Check sheet for the modelled part. Datum: model origin and axes. Units: mm. Face numbers are marked on the shaded views. A direction names the side the tool comes from. Coordinates: 2 decimals unless noted, no trailing zeros. Order: outer loops, then holes, each group sorted by start corner. A loop starts at its lowest first (then second) coordinate and runs counter-clockwise, first axis right, second up.
1. Draft check along X on the marked faces 1, 2 and 3. Enter one of: released by +X, released by -X, zero draft, split by the parting line, or undercut.
2. Cross-section at A-A (y = 0). Enter the section's corners in (x, z).
3. Thickness scan on line 1 (Y direction, x = 0, z = 8.25); line 2 (Y direction, x = 0.5, z = 1.25); line 3 (Z direction, x = 0.75, y = 1.9). Record the ranges inside material, lowest first.
4. Cross-section at B-B (x = 0). Enter the section's corners in (y, z).
5. Gauge pin test, flat ends, axial feed: pin 1 Ø1 at (y, z) = (-1, 4) entering from +X; pin 2 Ø0.6 at (y, z) = (-1.5, 0) entering from +X; pin 3 Ø0.5 at (x, y) = (0, 2) entering from -Z; pin 4 Ø1.6 at (x, y) = (0, 0) entering from +Z. Record the tip position at first contact, or that the pin passes through.
6. Cross-section at D-D (z = 9.5). Enter the section's corners in (x, y).
7. Cross-section at C-C (z = 1.5). Enter the section's corners in (x, y), then the cut area to 3 significant figures.
8. Set-up check for the marked faces 4 and 5: record each of +Z, -Z, +X, -X, +Y, -Y from which the full face is reachable in a straight line by a thin tool's end or side.
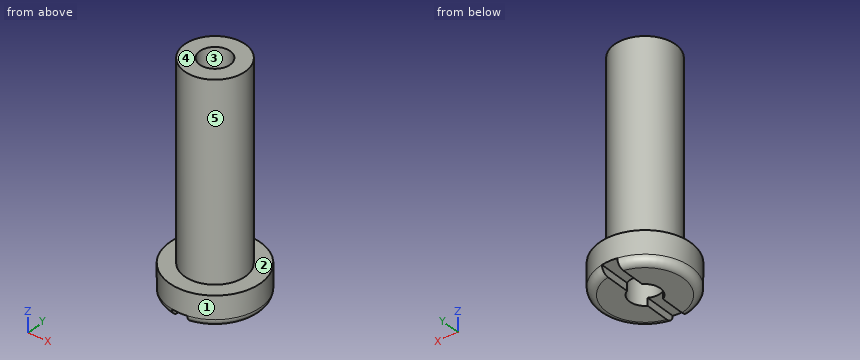
```python
from build123d import *

# Parameters (mm, degrees)
SKETCH1_R               = 3
BOSS_EXTRUDE1_DEPTH     = 2
FILLET1_R               = 0.5
SKETCH2_R               = 2
BOSS_EXTRUDE2_DEPTH     = 12.75
CUT_EXTRUDE1_DEPTH      = 16.348045478
CUT_EXTRUDE1_DEPTH_BACK = 16.348045478
SKETCH3_R               = 1
SKETCH4_W               = 1
SKETCH4_H               = 6
CUT_EXTRUDE3_DEPTH      = 0.5


with BuildPart() as part:
    # Sketch1 → Boss-Extrude1 (new body)
    with BuildSketch(Plane.XY):
        Circle(SKETCH1_R)
    extrude(amount=BOSS_EXTRUDE1_DEPTH)

    # Fillet1
    fillet1_edges = [part.edges().sort_by_distance(p)[0] for p in [
        (-3, 0, 0),
    ]]
    fillet(fillet1_edges, radius=FILLET1_R)

    # Sketch2 → Boss-Extrude2 (add)
    with BuildSketch(Plane.XY.offset(2)):
        Circle(SKETCH2_R)
    extrude(amount=BOSS_EXTRUDE2_DEPTH)

    # Sketch3 → Cut-Extrude1 (cut, two sides: drawn at the far end of the back side and taken through both)
    with BuildSketch(Plane(origin=(0, 0, 0), x_dir=(-1, 0, 0), z_dir=(0, 0, -1)).offset(-CUT_EXTRUDE1_DEPTH_BACK)):
        Circle(SKETCH3_R)
    extrude(amount=CUT_EXTRUDE1_DEPTH + CUT_EXTRUDE1_DEPTH_BACK, mode=Mode.SUBTRACT)

    # Sketch4 → Cut-Extrude3 (cut)
    with BuildSketch(Plane(origin=(0, 0, 0), x_dir=(-1, 0, 0), z_dir=(0, 0, -1))):
        Rectangle(SKETCH4_W, SKETCH4_H)
    extrude(amount=-CUT_EXTRUDE3_DEPTH, mode=Mode.SUBTRACT)


solid = part.part
```
Data:
1. face 1: split by the parting line
1. face 2: zero draft
1. face 3: undercut
2. outline: (-3, 0.5) arc R0.5 ccw to (-2.5, 0) - (-1, 0) - (-1, 14.75) - (-2, 14.75) - (-2, 2) - (-3, 2) - close; (1, 0) - (2.5, 0) arc R0.5 ccw to (3, 0.5) - (3, 2) - (2, 2) - (2, 14.75) - (1, 14.75) - close
3. line 1: y = -2 to -1, 1 to 2
3. line 2: y = -2.96 to -0.87, 0.87 to 2.96
3. line 3: z = 0 to 2
4. outline: (-3, 0.5) - (-1, 0.5) - (-1, 14.75) - (-2, 14.75) - (-2, 2) - (-3, 2) - close; (1, 0.5) - (3, 0.5) - (3, 2) - (2, 2) - (2, 14.75) - (1, 14.75) - close
5. pin 1: stops at x = 1.94
5. pin 2: stops at x = 2.61
5. pin 3: stops at z = 0.5
5. pin 4: passes through
6. outline: circle Ø4 at (0, 0); hole circle Ø2 at (0, 0)
7. outline: circle Ø6 at (0, 0); hole circle Ø2 at (0, 0)
7. area: 25.1 mm2
8. face 4: +Z, +X, -X, +Y, -Y
8. face 5: +Z
